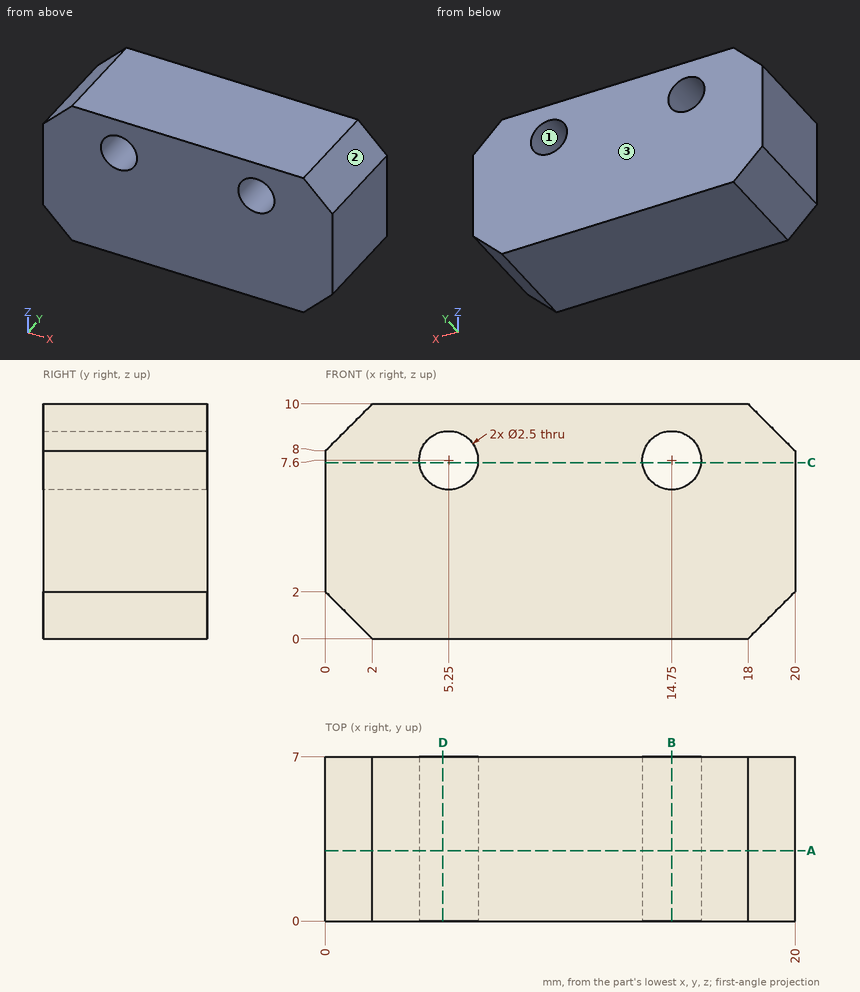
Can you work these out from the drawing? Everything is in mm from the part's minimum corner. Round coordinates to 2 decimals unless told otherwise and drop trailing zeros. Loops run counter-clockwise (first coordinate to the right, second up) from the corner with the lowest first, then second, coordinate; pieces in that order, holes last. Notation, with made-up numbers: (-10, 40) - (32, 40) arc R19 ccw to (32, 69) - close; hole circle Ø9 at (50, -23). An arc over 180 degrees is marked (long way). Write item = value, one per line. Start each with the question number.
(1) If we section it at D-D (x = 5): Please give me the cut outline in (y, z).
(2) If we mould it in two halves opening along Z, with no side actions, what happens to the marked faces 1, 2 and 3? For each: released by +Z, released by -Z, zero draft, split by the parting line, or undercut.
(3) If we section it at C-C (z = 7.5): Please give me the cut outline in (x, y).
(4) If we section it at A-A (y = 3): Please give me the cut outline in (x, z).
(5) If we section it at B-B (x = 14.75): Please give me the cut outline in (y, z), and give its area (3 significant figures).
(6) If I drill on probe 1 along X at (y, z) = (1.75, 7.6); probe 2 along Z at (x, y) = (6.25, 2); probe 3 along Z at (x, y) = (1.25, 2.75), over which ranges is the centre line in solid material (lowest first)? Write a range as [from, to].
Ans:
q1.outline = (0, 0) - (7, 0) - (7, 6.38) - (0, 6.38) - close; (0, 8.82) - (7, 8.82) - (7, 10) - (0, 10) - close
q2.face_1 = undercut
q2.face_2 = released by +Z
q2.face_3 = zero draft
q3.outline = (0, 0) - (4, 0) - (4, 7) - (0, 7) - close; (6.5, 0) - (13.5, 0) - (13.5, 7) - (6.5, 7) - close; (16, 0) - (20, 0) - (20, 7) - (16, 7) - close
q4.outline = (0, 2) - (2, 0) - (18, 0) - (20, 2) - (20, 8) - (18, 10) - (2, 10) - (0, 8) - close; hole circle Ø2.5 at (5.25, 7.6); hole circle Ø2.5 at (14.75, 7.6)
q5.outline = (0, 0) - (7, 0) - (7, 6.35) - (0, 6.35) - close; (0, 8.85) - (7, 8.85) - (7, 10) - (0, 10) - close
q5.area = 52.5 mm²
q6.probe_1 = [0, 4], [6.5, 13.5], [16, 20]
q6.probe_2 = [0, 6.85], [8.35, 10]
q6.probe_3 = [0.75, 9.25]
